Autodesk Inventor part; units mm, degrees
ref_plane "YZ Plane" through (0, 0, 0) normal (1, 0, 0) x (0, 1, 0)
ref_plane "XZ Plane" through (0, 0, 0) normal (0, 1, 0) x (-1, 0, 0)
ref_plane "XY Plane" through (0, 0, 0) normal (0, 0, 1) x (1, 0, 0)
ref_plane "Arbeitsebene1" through (-22.9558, 17.7058, 46.5) normal (0, 0, -1) x (-1, 0, 0)
sketch "Skizze1" plane through (0, 0, 0) normal (0, 0, 1) x (1, 0, 0)
  circle A0 centre (0, 0) radius 3.55
  line L0 (-14.5, 14.5) -> (4.5, 14.5)
  line L1 (4.5, 14.5) -> (4.5, -4.5)
  line L2 (4.5, -4.5) -> (-14.5, -4.5)
  line L3 (-14.5, -4.5) -> (-14.5, 14.5)
  dimension "d0" = 7.1
  dimension "d1" = 19
  dimension "d2" = 19
  dimension "d3" = 4.5
  dimension "d4" = 4.5
extrude "Extrusion1" add sketch "Skizze1" along normal blind 3
sketch "Skizze2" plane through (0, 0, 0) normal (0, 0, -1) x (-1, 0, 0)
  line L0 (14.5, 14.5) -> (14.5, -4.5)
  line L1 (-4.5, 14.5) -> (14.5, 14.5)
  circle A0 centre (0, 0) radius 3.55
  line L2 (14.5, -4.5) -> (-4.5, -4.5)
  line L3 (-4.5, -4.5) -> (-4.5, 14.5)
  line L4 (-4.5, 14.5) -> (14.5, 14.5)
  line L5 (14.5, 14.5) -> (14.5, -4.5)
  line L6 (14.5, -4.5) -> (-4.5, -4.5)
  line L7 (-4.5, -4.5) -> (-4.5, 14.5)
  line L8 (-3, -4.5) -> (-3, 13)
  line L9 (-3, 13) -> (13, 13)
  line L10 (13, 13) -> (13, -3)
  line L11 (13, -3) -> (-0.4, -3)
  line L12 (-4.5, -4.5) -> (4.5, -4.5)
  line L13 (4.5, -4.5) -> (4.5, 4.5)
  line L14 (4.5, 4.5) -> (-4.5, 4.5)
  line L15 (-4.5, 4.5) -> (-4.5, -4.5)
  line L16 (-3, 13) -> (13, 13)
  line L17 (13, 13) -> (13, 14.5)
  line L18 (13, 14.5) -> (-3, 14.5)
  line L19 (-3, 14.5) -> (-3, 13)
  point P0 (4.5, -3)
  point P1 (4.5, -4.5)
  point P2 (13, 14.5)
  point P3 (-4.5, 4.5)
  point P4 (-3, 4.5)
  dimension "d13" = 1.5
  dimension "d14" = 9
  dimension "d15" = 9
extrude "Extrusion2" add sketch "Skizze2" along normal blind 15 contours L0 L2 L13 L11 L10 L17 L1 | L19 L8 L14 L3 L1
sketch "Skizze3" plane through (0, 0, -15) normal (0, 0, -1) x (-1, 0, 0)
  line L0 (-4.5, 14.5) -> (14.5, 14.5)
  line L1 (14.5, 14.5) -> (14.5, -4.5)
  circle A0 centre (0, 0) radius 3.55
  line L2 (14.5, -4.5) -> (-4.5, -4.5)
  line L3 (-4.5, -4.5) -> (-4.5, 14.5)
extrude "Extrusion3" add sketch "Skizze3" along normal blind 3
sketch "Skizze4" plane through (0, 0, 3) normal (0, 0, 1) x (1, 0, 0)
  line L0 (-14.5, -4.5) -> (4.5, -4.5)
  line L1 (4.5, -4.5) -> (4.5, 14.5)
  line L2 (4.5, 14.5) -> (-14.5, 14.5)
  line L3 (-14.5, 14.5) -> (-14.5, -4.5)
  circle A0 centre (0, 0) radius 3.55
  line L4 (4.5, -4.5) -> (-5.5, -4.5)
  line L5 (-5.5, -4.5) -> (-5.5, 5.5)
  line L6 (-5.5, 5.5) -> (4.5, 5.5)
  line L7 (4.5, 5.5) -> (4.5, -4.5)
  dimension "d16" = 10
  dimension "d17" = 10
extrude "Extrusion4" add sketch "Skizze4" along normal blind 5 contours L5 L6 L1 L0
sketch "Skizze5" plane through (0, 0, -18) normal (0, 0, -1) x (-1, 0, 0)
  line L0 (-4.5, -4.5) -> (14.5, -4.5)
  line L1 (14.5, -4.5) -> (14.5, 14.5)
  line L2 (14.5, 14.5) -> (-4.5, 14.5)
  line L3 (-4.5, 14.5) -> (-4.5, -4.5)
  circle A0 centre (0, 0) radius 3.55
  line L4 (-4.5, -4.5) -> (5.5, -4.5)
  line L5 (5.5, -4.5) -> (5.5, 5.5)
  line L6 (5.5, 5.5) -> (-4.5, 5.5)
  line L7 (-4.5, 5.5) -> (-4.5, -4.5)
  dimension "d20" = 10
  dimension "d21" = 10
extrude "Extrusion5" add sketch "Skizze5" along normal blind 5 contours L3 L6 L5 L0
chamfer "Fasen1" distance 2 angle 45 8 edges at (-0.5, 5.5, 3) (-5.5, 0.5, 3) (-14.5, 5, 3) (-13, 5, 0) (-13, 5, -15) (-14.5, 5, -18) (-5.5, 0.5, -18) (-0.5, 5.5, -18)
properties part number "HolisheetCageSampleWater"
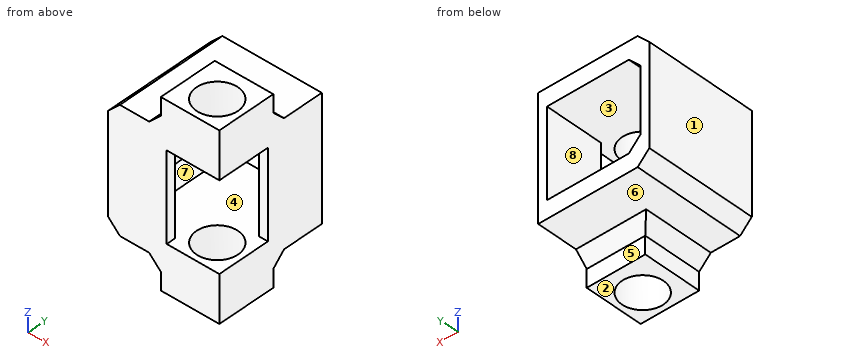
For this review, take the finished solid that the model builds, in its own axes (mm). Face numbers are marked on the shaded views. A direction names the side the tool comes from. Round coordinates to 2 decimals unless told otherwise and drop trailing zeros. Loops run counter-clockwise (first coordinate to the right, second up) from the corner with the lowest first, then second, coordinate; pieces in that order, holes last. Notation, with made-up numbers: (59, 14.25) - (112, 14.25) arc R33 cw to (112, 42.25) - close; hole circle Ø9 at (35.5, 48). An arc over 180 degrees is marked (long way). Answer as CSV lines item,"result".
(1) Tool access review of the marked faces 5, 6, 7 and 8: name each direction out of +Z, -Z, +X, -X, +Y, -Y from which nothing blocks a thin tool from reaching the whole face with its end or side.
Checked values:
face 5,"-Z, +X, -X, +Y"
face 6,"-Z, -X, +Y"
face 7,"+Y"
face 8,"+Y, -Y"
(2) Mouldability with a two-part tool opening along X and no side actions: class the marked faces 1, 2, 3 and 4 as +X half, -X half, draft (parallel to the pull), parting line (faces both ways), or undercut.
Checked values:
face 1,"-X half"
face 2,"draft"
face 3,"undercut"
face 4,"undercut"
(3) Consider section A-A on x = 0. Give the boundary of the cut face in (y, z).
Checked values:
outline,"(-4.5, -23) - (-3.55, -23) - (-3.55, -15) - (-4.5, -15) - close; (-4.5, 0) - (-3.55, 0) - (-3.55, 8) - (-4.5, 8) - close; (3.55, -23) - (5.5, -23) - (5.5, -20) - (7.5, -18) - (14.5, -18) - (14.5, -15) - (3.55, -15) - close; (3.55, 0) - (14.5, 0) - (14.5, 3) - (7.5, 3) - (5.5, 5) - (5.5, 8) - (3.55, 8) - close"
(4) Insertion check: P1, Ø4, axis at x = -9.5, z = -6.5, coming from the +Y side; P2, Ø1.2, axis at x = 3.5, z = -5.5, coming from the -Y side; P3, Ø0.8, axis at y = -4, z = -5, coming from the +X side. Each pin has a flat end and moves straight along its axis. Give the tip position at first contact, or say it passes through.
Checked values:
P1,"stops at y = -3"
P2,"stops at y = 4.5"
P3,"stops at x = -4.5"
(5) Consider section B-B on y = 0. Give the boundary of the cut face in (x, z).
Checked values:
outline,"(-14.5, -16) - (-12.5, -18) - (-7.5, -18) - (-5.5, -20) - (-5.5, -23) - (-3.55, -23) - (-3.55, -15) - (-11, -15) - (-13, -13) - (-13, -2) - (-11, 0) - (-3.55, 0) - (-3.55, 8) - (-5.5, 8) - (-5.5, 5) - (-7.5, 3) - (-12.5, 3) - (-14.5, 1) - close; (3.55, -23) - (4.5, -23) - (4.5, -15) - (3.55, -15) - close; (3.55, 0) - (4.5, 0) - (4.5, 8) - (3.55, 8) - close"
(6) Consider section D-D on x = -6.75. Give the boundary of the cut face in (y, z), then the cut area to 3 significant figures.
Checked values:
outline,"(-4.5, -18.75) - (6.75, -18.75) - (7.5, -18) - (14.5, -18) - (14.5, -15) - (-3, -15) - (-3, 0) - (14.5, 0) - (14.5, 3) - (7.5, 3) - (6.75, 3.75) - (-4.5, 3.75) - close"
area,"154 mm2"
(7) Wall thickness on line 1 (Z direction, x = -5.75, y = 10.5); line 2 (X direction, y = 13.5, z = -13); line 3 (Y direction, x = 0, z = -20.25): over which ranges is each line inside the solid? List them lowest first.
Checked values:
line 1,"z = -18 to -15, 0 to 3"
line 2,"x = -14.5 to -13, 3 to 4.5"
line 3,"y = -4.5 to -3.55, 3.55 to 5.5"
(8) Consider section C-C on z = -9. Give the boundary of the cut face in (x, y).
Checked values:
outline,"(-14.5, -4.5) - (-4.5, -4.5) - (-4.5, -3) - (-13, -3) - (-13, 14.5) - (-14.5, 14.5) - close; (3, 4.5) - (4.5, 4.5) - (4.5, 14.5) - (3, 14.5) - close"
